Geometry: see drawing. Coordinates: mm, zero at the bounding-box minimum. Round coordinates to 2 decimals unless told otherwise and drop trailing zeros. Write each loop counter-clockwise with the first axis right and the second up, starting at its lowest first coordinate (ties: lowest second). Pieces come first, ordered by that corner, then holes.
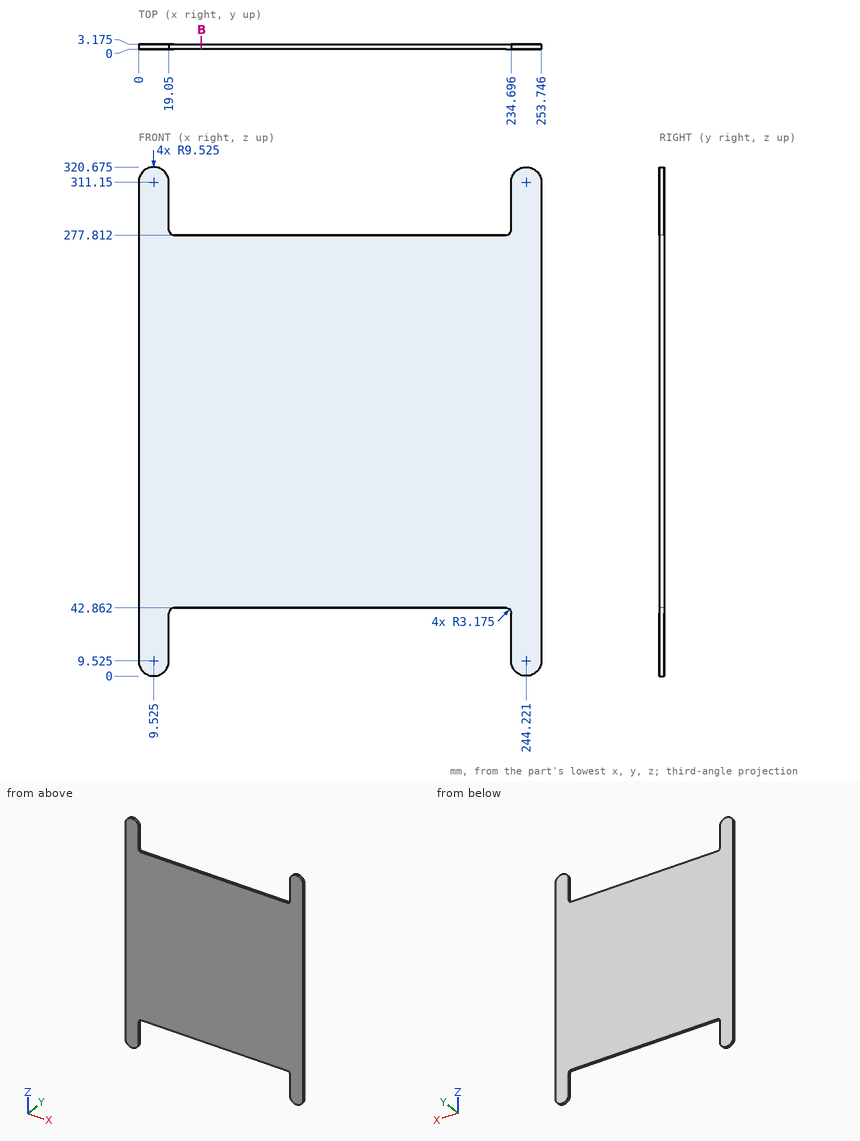
Q1. Line query: line 1 (X direction, y = 2.2, z = 285); line 2 (Z direction, x = 123.5, y = 0.4); line 3 (X direction, y = 1, z = 279.5) (1 decimal). Output: solid intervals per line, ascending.
Q2. Pin query (flat end, axial travel): P1, Ø1, axis at x = 125, y = 2.5, coming from the +Z side. Return the tip coordinate at first contact, or that it passes through.
Q3. Section query B-B, the plane x = 39.5. Output: boundary loops of the cut face in (y, z) (1 decimal).
Filled in:
1. line 1: x = 0 to 19.05, 234.7 to 253.75
1. line 2: z = 42.86 to 277.81
1. line 3: x = 0 to 19.4, 234.3 to 253.7
2. P1: stops at z = 277.81
3. outline: (0, 42.9) - (3.2, 42.9) - (3.2, 277.8) - (0, 277.8) - close
